Check sheet for the modelled part. Datum: model origin and axes. Units: mm. Face numbers are marked on the shaded views. A direction names the side the tool comes from. Coordinates: 2 decimals unless noted, no trailing zeros. Write each loop counter-clockwise with the first axis right and the second up, starting at its lowest first coordinate (ties: lowest second). Pieces come first, ordered by that corner, then holes. Notation, with made-up numbers: (39.5, 69) -> (97.5, 69) arc R18 cw to (97.5, 90) -> close; hole circle Ø2 at (-23.5, 65.25). An arc over 180 degrees is marked (long way). One line per item, written item: value. Start each with the question number.
1) Sectioned sample at D-D on x = 18. Enter the section's corners in (y, z).
2) Set-up check for the marked faces 3 and 4: record each of +Z, -Z, +X, -X, +Y, -Y from which the full face is reachable in a straight line by a thin tool's end or side.
3) Sectioned sample at C-C on z = 22. Enter the section's corners in (x, y), plus the area to 3 significant figures.
4) Draft check along X on the marked faces 1 and 2. Enter one of: +X half, -X half, draft (parallel to the pull), parting line (faces both ways), or undercut.
5) Gauge pin test, flat ends, axial feed: P1, Ø0.8, axis at y = 4.5, z = -82, coming from the -X side; P2, Ø1.1, axis at y = 4.5, z = -35, coming from the +X side; P3, Ø4, axis at x = 24, z = -39.5, coming from the +Y side; P4, Ø0.5, axis at y = 4.5, z = 30.5, coming from the +X side. Record the tip position at first contact, or that the pin passes through.
6) Scan lines: line 1 along X through (y, z) = (4.1, -37) (3 decimals); line 2 along Z through (x, y) = (13, 4.8); line 3 along Y through (x, z) = (-49.5, 68.5). Record each from-to range of solid material in increasing order. Write a range as [from, to].
7) Sectioned sample at A-A on y = 1.2. Enter the section's corners in (x, z).
8) Sectioned sample at B-B on x = -40. Enter the section's corners in (y, z), plus the area to 3 significant figures.
```python
from build123d import *

# Parameters (mm, degrees)
SKETCH1_W           = 90
SKETCH1_H           = 190
BOSS_EXTRUDE1_DEPTH = 5
SKETCH2_W           = 10
SKETCH2_H           = 30
BOSS_EXTRUDE2_DEPTH = 5
CHAMFER1_SIZE       = 2
SKETCH3_W           = 16
SKETCH3_H           = 34
CUT_EXTRUDE1_DEPTH  = 50
SKETCH4_W           = 90
SKETCH4_H           = 42
CUT_EXTRUDE2_DEPTH  = 1
CUT_EXTRUDE5_START  = 5
SKETCH5_W           = 6
SKETCH5_H           = 3
CUT_EXTRUDE5_DEPTH  = 1
SKETCH6_W           = 6.2
SKETCH6_H           = 3.2
CUT_EXTRUDE6_DEPTH  = 1
SKETCH7_W           = 15.1
SKETCH7_H           = 89.916335477
CUT_EXTRUDE7_DEPTH  = 1
CUT_EXTRUDE8_DEPTH  = 1


with BuildPart() as part:
    # Sketch1 → Boss-Extrude1 (new body)
    with BuildSketch(Plane(origin=(0, 0, 0), x_dir=(1, 0, 0), z_dir=(0, 1, 0))):
        Rectangle(SKETCH1_W, SKETCH1_H)
    extrude(amount=BOSS_EXTRUDE1_DEPTH)

    # Sketch2 → Boss-Extrude2 (add)
    with BuildSketch(Plane(origin=(0, 0, 0), x_dir=(1, 0, 0), z_dir=(0, 1, 0))):
        with Locations((-50, -80)):
            Rectangle(SKETCH2_W, SKETCH2_H)
        with Locations((50, -80)):
            Rectangle(SKETCH2_W, SKETCH2_H)
    extrude(amount=BOSS_EXTRUDE2_DEPTH)

    # Chamfer1
    chamfer1_edges = [part.edges().sort_by_distance(p)[0] for p in [
        (-55, 2.5, 65),
        (-55, 2.5, 95),
        (55, 2.5, 95),
        (55, 2.5, 65),
    ]]
    chamfer(chamfer1_edges, length=CHAMFER1_SIZE)

    # Sketch3 → Cut-Extrude1 (cut)
    with BuildSketch(Plane(origin=(0, 5, 0), x_dir=(1, 0, 0), z_dir=(0, 1, 0))):
        with Locations((-25, -78)):
            Rectangle(SKETCH3_W, SKETCH3_H)
    extrude(amount=-CUT_EXTRUDE1_DEPTH, mode=Mode.SUBTRACT)

    # Sketch4 → Cut-Extrude2 (cut)
    with BuildSketch(Plane(origin=(0, 5, 0), x_dir=(1, 0, 0), z_dir=(0, 1, 0))):
        with Locations((0, 59.159820088)):
            Rectangle(SKETCH4_W, SKETCH4_H)
    extrude(amount=-CUT_EXTRUDE2_DEPTH, mode=Mode.SUBTRACT)

    # Sketch5 → Cut-Extrude5 (cut)
    with BuildSketch(Plane(origin=(0, 0, 0), x_dir=(1, 0, 0), z_dir=(0, 1, 0)).offset(CUT_EXTRUDE5_START)):
        with Locations((-11.605, 35.659820088)):
            Rectangle(SKETCH5_W, SKETCH5_H)
        with Locations((-11.605, 82.659820088)):
            Rectangle(SKETCH5_W, SKETCH5_H)
        with Locations((11.605, 35.659820088)):
            Rectangle(SKETCH5_W, SKETCH5_H)
        with Locations((11.605, 82.659820088)):
            Rectangle(SKETCH5_W, SKETCH5_H)
    extrude(amount=-CUT_EXTRUDE5_DEPTH, mode=Mode.SUBTRACT)

    # Sketch6 → Cut-Extrude6 (cut)
    with BuildSketch(Plane(origin=(0, 5, 0), x_dir=(1, 0, 0), z_dir=(0, 1, 0))):
        with Locations((11.605, 82.659820088)):
            Rectangle(SKETCH6_W, SKETCH6_H)
        with Locations((-11.605, 82.659820088)):
            Rectangle(SKETCH6_W, SKETCH6_H)
    extrude(amount=-CUT_EXTRUDE6_DEPTH, mode=Mode.SUBTRACT)

    # Sketch7 → Cut-Extrude7 (cut)
    with BuildSketch(Plane(origin=(0, 5, 0), x_dir=(1, 0, 0), z_dir=(0, 1, 0))):
        with Locations((37.45, -15.495273531)):
            Rectangle(SKETCH7_W, SKETCH7_H)
        with Locations((0.16773297, -15.495273531)):
            Rectangle(SKETCH7_W, SKETCH7_H)
    extrude(amount=-CUT_EXTRUDE7_DEPTH, mode=Mode.SUBTRACT)

    # Sketch8 → Cut-Extrude8 (cut)
    with BuildSketch(Plane(origin=(0, 5, 0), x_dir=(1, 0, 0), z_dir=(0, 1, 0))):
        Polygon((-34.9, -70.1), (-45.958578644, -70.1), (-47.9, -72.041421356), (-47.9, -87.958578644), (-45.958578644, -89.9), (-34.9, -89.9), (-34.9, -95.1), (-53.041421356, -95.1), (-55.1, -93.041421356), (-55.1, -66.958578644), (-53.041421356, -64.9), (-34.9, -64.9), align=None)
    cut_extrude8 = extrude(amount=-CUT_EXTRUDE8_DEPTH, mode=Mode.SUBTRACT)

    # Mirror1: Cut-Extrude8 across plane
    add(cut_extrude8.mirror(Plane(origin=(0, 0, 0), x_dir=(0, 0, 1), z_dir=(1, 0, 0))), mode=Mode.SUBTRACT)


solid = part.part
```
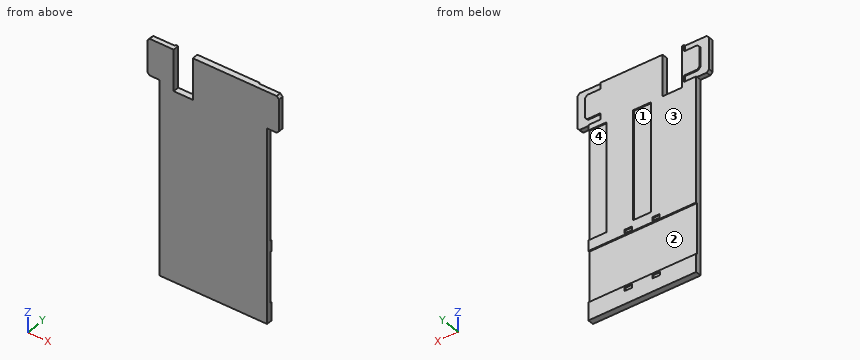
Answers:
1. outline: (0, -95) -> (5, -95) -> (5, -80.16) -> (4, -80.16) -> (4, -38.16) -> (5, -38.16) -> (5, 95) -> (0, 95) -> close
2. face 3: +Z, -Z, +X, -X, +Y
2. face 4: +X, +Y
3. outline: (-45, 0) -> (45, 0) -> (45, 4) -> (29.9, 4) -> (29.9, 5) -> (7.72, 5) -> (7.72, 4) -> (-7.38, 4) -> (-7.38, 5) -> (-45, 5) -> close
3. area: 420 mm2
4. face 1: undercut
4. face 2: draft
5. P1: stops at x = -45
5. P2: stops at x = 45
5. P3: stops at y = 5
5. P4: stops at x = 29.9
6. line 1: x = [-45, -14.605], [-8.605, 8.605], [14.605, 45]
6. line 2: z = [-95, -84.26], [-81.06, -80.16], [-38.16, -37.16], [-34.16, 95]
6. line 3: y = [0, 4]
7. outline: (-55, 67) -> (-53, 65) -> (-45, 65) -> (-45, -95) -> (45, -95) -> (45, 65) -> (53, 65) -> (55, 67) -> (55, 93) -> (53, 95) -> (-17, 95) -> (-17, 61) -> (-33, 61) -> (-33, 95) -> (-53, 95) -> (-55, 93) -> close
8. outline: (0, -95) -> (5, -95) -> (5, -80.16) -> (4, -80.16) -> (4, -38.16) -> (5, -38.16) -> (5, 64.9) -> (4, 64.9) -> (4, 70.1) -> (5, 70.1) -> (5, 89.9) -> (4, 89.9) -> (4, 95) -> (0, 95) -> close
8. area: 898 mm2
